from build123d import *

# Parameters (mm, degrees)
F0_R        = 2
F1_DEPTH    = 6
F2_DEPTH    = 93
F4_DEPTH    = 25
F3_R        = 1.75
F5_DEPTH    = 4.001
F6_W        = 73
F6_H        = 161
F6_R        = 2.25
F7_DEPTH    = 4.001
F8_T4_DEPTH = 4
F9_R        = 13


# Not quite as in the source:
# - a fillet or chamfer that OpenCascade refuses, or shapes differently, is made with other operations: its cross-section is extruded or revolved along the edge and cut away or added


with BuildPart() as f1:
    # F0 (on Right) → F1 (new body)
    with BuildSketch(Plane.YZ):
        Polygon((-4.3, 0), (-34.3, 0), (-34.3, 52), (-34.3, 64), (-34.3, 169), (-34.3, 181), (-38.3, 181), (-38.3, -4), (-4.3, -4), align=None)
        with BuildLine():
            Line((-34.3, 181), (-34.3, 169))
            Line((-34.3, 169), (0, 169))
            ThreePointArc((0, 169), (-6, 174.9999999833), (-3.34e-08, 181))
            Line((-3.34e-08, 181), (-34.3, 181))
        make_face()
        with BuildLine():
            Line((-34.3, 64), (-34.3, 52))
            Line((-34.3, 52), (-5.41e-08, 52))
            ThreePointArc((-5.41e-08, 52), (-6, 58.0000000477), (4.13e-08, 64))
            Line((4.13e-08, 64), (-34.3, 64))
        make_face()
        with BuildLine():
            ThreePointArc((-3.34e-08, 181), (-6, 174.9999999833), (0, 169))
            ThreePointArc((0, 169), (4.2426406871, 170.7573593129), (6, 175))
            ThreePointArc((6, 175), (4.2426406753, 179.2426406989), (-3.34e-08, 181))
        make_face()
        with Locations((0, 175)):
            Circle(F0_R, mode=Mode.SUBTRACT)
        with BuildLine():
            ThreePointArc((4.13e-08, 64), (-6, 58.0000000477), (-5.41e-08, 52))
            ThreePointArc((-5.41e-08, 52), (4.242640668, 53.7573592937), (6, 58))
            ThreePointArc((6, 58), (4.2426407017, 62.2426406725), (4.13e-08, 64))
        make_face()
        with Locations((0, 58)):
            Circle(F0_R, mode=Mode.SUBTRACT)
    extrude(amount=F1_DEPTH)

    # F0 (on Right) → F2 (join)
    with BuildSketch(Plane.YZ):
        Polygon((-4.3, 0), (-34.3, 0), (-34.3, 52), (-34.3, 64), (-34.3, 169), (-34.3, 181), (-38.3, 181), (-38.3, -4), (-4.3, -4), align=None)
    extrude(amount=-F2_DEPTH)

    # F0 (on Right) → F4 (join)
    with BuildSketch(Plane.YZ):
        Polygon((-4.3, 0), (-34.3, 0), (-34.3, 52), (-34.3, 64), (-34.3, 169), (-34.3, 181), (-38.3, 181), (-38.3, -4), (-4.3, -4), align=None)
    extrude(amount=-F4_DEPTH)

    # F3 (on face) → F5 (cut, through all)
    with BuildSketch(Plane.XY):
        with Locations((-89, -27.8)):
            Circle(F3_R)
        with Locations((-69, -27.8)):
            Circle(F3_R)
    extrude(amount=-F5_DEPTH, mode=Mode.SUBTRACT)

    # F6 (on face) → F7 (cut, through all)
    with BuildSketch(Plane(origin=(0, -34.3, 0), x_dir=(-1, 0, 0), z_dir=(0, 1, 0))):
        with Locations((56.5, 100.5)):
            Rectangle(F6_W, F6_H)
        with BuildLine():
            ThreePointArc((20, 2), (24.9497474683, 4.0502525317), (27, 9))
            ThreePointArc((27, 9), (24.9497474683, 13.9497474683), (20, 16))
            ThreePointArc((20, 16), (13, 9), (20, 2))
        make_face()
        with BuildLine():
            ThreePointArc((34, 2), (29.0502525317, 4.0502525317), (27, 9))
            ThreePointArc((27, 9), (24.9497474683, 4.0502525317), (20, 2))
            Line((20, 2), (34, 2))
        make_face()
        with BuildLine():
            ThreePointArc((20, 16), (24.9497474683, 13.9497474683), (27, 9))
            ThreePointArc((27, 9), (29.0502525317, 13.9497474683), (34, 16))
            Line((34, 16), (20, 16))
        make_face()
        with BuildLine():
            ThreePointArc((34, 16), (29.0502525317, 13.9497474683), (27, 9))
            ThreePointArc((27, 9), (29.0502525317, 4.0502525317), (34, 2))
            ThreePointArc((34, 2), (38.9497474683, 4.0502525317), (41, 9))
            ThreePointArc((41, 9), (38.9497474683, 13.9497474683), (34, 16))
        make_face()
        with Locations((7.5, 166)):
            Circle(F6_R)
        with Locations((7.5, 58)):
            Circle(F6_R)
        with Locations((55, 10)):
            Circle(F6_R)
    extrude(amount=-F7_DEPTH, mode=Mode.SUBTRACT)

    # F8: fillet of radius 73.1506709399 on 1 edges, made by hand


with BuildPart() as f8_tool2:
    # F8_s3 → F8_t4 (new body)
    with BuildSketch(Plane.XZ.offset(34.3)):
        with BuildLine():
            ThreePointArc((-93.1506709399, 20), (-41.42533547, 41.42533547), (-20, 93.1506709399))
            Line((-20, 93.1506709399), (-20, 20))
            Line((-20, 20), (-93.1506709399, 20))
        make_face()
    extrude(amount=F8_T4_DEPTH)

    split(bisect_by=Plane.YZ.offset(-93), keep=Keep.TOP)


with BuildPart() as f1_1:
    add(f1.part)

    # F8_t1: union F8_tool2
    add(f8_tool2.part)

    # F9
    f9_edges = [f1_1.edges().sort_by_distance(p)[0] for p in [
        (-20, -36.3, 181),
        (-93, -36.3, 20.000155),
    ]]
    fillet(f9_edges, radius=F9_R)


solid = f1_1.part
Could you check a few things on this model? Use its own coordinates, in mm. A direction names the side the tool comes from. Round coordinates to 2 decimals unless told otherwise and drop trailing zeros. Order: outer loops, then holes, each group sorted by start corner. A loop starts at its lowest first (then second) coordinate and runs counter-clockwise, first axis right, second up.
Q1. Which directions (+Z, -Z, +X, -X, +Y, -Y) give clear straight access to the entire face, cutting with the end or side of a thin tool? Please do faces 1 (the face through (3, -17, 64)), 2 (the face through (-20, -36, 130)), 3 (the face through (-27, -36, 2)), 4 (the face through (0, -14, 175)), 5 (the face through (6, -36, 103)).
Geometry says:
face 1: +X, -X, +Y
face 2: +Z, -X, +Y, -Y
face 3: +Y, -Y
face 4: +Z, -X, +Y
face 5: +Z, -Z, +X, +Y, -Y
Q2. I'm going to push flat-ended pins straight in: P1, Ø1.2, axis at x = -48.5, z = -2.5, coming from the +Y side; P2, Ø6, axis at x = -33.5, y = -12, coming from the +Z side; P3, Ø9.5, axis at y = -18.5, z = 55.5, coming from the -X side. Where does each tip first touch, or does it pass through?
Geometry says:
P1: stops at y = -4.3
P2: stops at z = 0
P3: stops at x = 0
Q3. Imagine slicing it at D-D, the plane x = -2.5. List the corners of the cut face in (y, z) for me, then the cut area to 3 significant figures.
Geometry says:
outline: (-38.3, -4) - (-4.3, -4) - (-4.3, 0) - (-34.3, 0) - (-34.3, 181) - (-38.3, 181) - close
area: 860 mm2
Q4. Please list where these lines run through material, in increasing order: probe 1 along Z at (x, y) = (-7.5, -35.9); probe 2 along Y at (x, z) = (4.6, 175); probe 3 along Y at (x, z) = (-69, -1.9).
Geometry says:
probe 1: z = -4 to 55.75, 60.25 to 163.75, 168.25 to 180.99
probe 2: y = -38.3 to -2, 2 to 6
probe 3: y = -38.3 to -29.55, -26.05 to -4.3
Q5. Imagine slicing it at C-C, the plane x = -69. List the corners of the cut face in (y, z) for me.
Geometry says:
outline: (-38.3, -4) - (-29.55, -4) - (-29.55, 0) - (-34.3, 0) - (-34.3, 24.1) - (-38.3, 24.1) - close; (-26.05, -4) - (-4.3, -4) - (-4.3, 0) - (-26.05, 0) - close
Q6. Imagine slicing it at A-A, the plane y = -7. List the corners of the cut face in (x, z) for me, then the cut area to 3 significant figures.
Geometry says:
outline: (-93, -4) - (6, -4) - (6, 0) - (-93, 0) - close; (0, 52) - (6, 52) - (6, 64) - (0, 64) - close; (0, 169) - (6, 169) - (6, 181) - (0, 181) - close
area: 540 mm2
Q7. Thinking about a two-plate mould opening in Z: for faces 6 (the face through (3, -17, 169)), 7 (the face through (-16.091, -36.328, 177.293)), 8 (the face through (-93, -25, -1)), which applies, released by +Z, released by -Z, zero draft, split by the parting line, or undercut?
Geometry says:
face 6: undercut
face 7: released by +Z
face 8: zero draft
Q8. Imagine slicing it at B-B, the plane y = -27.8. List the corners of the cut face in (x, z) for me.
Geometry says:
outline: (-93, -4) - (-90.75, -4) - (-90.75, 0) - (-93, 0) - close; (-87.25, -4) - (-70.75, -4) - (-70.75, 0) - (-87.25, 0) - close; (-67.25, -4) - (6, -4) - (6, 0) - (-67.25, 0) - close; (0, 52) - (6, 52) - (6, 64) - (0, 64) - close; (0, 169) - (6, 169) - (6, 181) - (0, 181) - close
